```python
from build123d import *

# Parameters (mm, degrees)
SKETCH_1_R      = 1.6
SKETCH_1_R_2    = 20
SKETCH_1_R_3    = 2.1
EXTRUDE_1_DEPTH = 2
FILLET_1_R      = 3


with BuildPart() as part:
    # 草图1 → 凸台-拉伸1 (new body)
    with BuildSketch(Plane(origin=(0, 0, 0), x_dir=(1, 0, 0), z_dir=(0, 1, 0))):
        Polygon((52, 16), (-52, 16), (-52, -16), (-27.5, -16), (-27.5, -44), (27.5, -44), (27.5, -16), (52, -16), align=None)
        with Locations(Location((25, -41.5, 0), (0, 0, 270))):
            Circle(SKETCH_1_R, mode=Mode.SUBTRACT)
        with Locations(Location((-25, -41.5, 0), (0, 0, 270))):
            Circle(SKETCH_1_R, mode=Mode.SUBTRACT)
        with Locations(Location((0, -16.5, 0), (0, 0, 270))):
            Circle(SKETCH_1_R_2, mode=Mode.SUBTRACT)
        with Locations(Location((-49.1, -12.5, 0), (0, 0, 270))):
            Circle(SKETCH_1_R_3, mode=Mode.SUBTRACT)
        with Locations(Location((-49.1, 12.5, 0), (0, 0, 270))):
            Circle(SKETCH_1_R_3, mode=Mode.SUBTRACT)
        with Locations(Location((-25, 8.5, 0), (0, 0, 270))):
            Circle(SKETCH_1_R, mode=Mode.SUBTRACT)
        with Locations(Location((49.1, -12.5, 0), (0, 0, 270))):
            Circle(SKETCH_1_R_3, mode=Mode.SUBTRACT)
        with Locations(Location((25, 8.5, 0), (0, 0, 270))):
            Circle(SKETCH_1_R, mode=Mode.SUBTRACT)
        with Locations(Location((49.1, 12.5, 0), (0, 0, 270))):
            Circle(SKETCH_1_R_3, mode=Mode.SUBTRACT)
    extrude(amount=EXTRUDE_1_DEPTH)

    # 圆角1
    fillet_1_edges = [part.edges().sort_by_distance(p)[0] for p in [
        (27.5, 1, 44),
        (-27.5, 1, 44),
        (-27.5, 1, 16),
        (-52, 1, 16),
        (-52, 1, -16),
        (52, 1, -16),
        (52, 1, 16),
        (27.5, 1, 16),
    ]]
    fillet(fillet_1_edges, radius=FILLET_1_R)


solid = part.part
```
Could you check a few things on this model? Use its own coordinates, in mm. A direction names the side the tool comes from. Round coordinates to 2 decimals unless told otherwise and drop trailing zeros. Loops run counter-clockwise (first coordinate to the right, second up) from the corner with the lowest first, then second, coordinate; pieces in that order, holes last. Notation, with made-up numbers: (72.25, 21) - (98.25, 21) arc R21 cw to (98.25, 42) - close; hole circle Ø11 at (43.5, 36). An arc over 180 degrees is marked (long way). Answer in a Markdown table with one row per item. Add a question column.
(1) If we section it at C-C (y = 0.8): State how many separate pieces and enclosed holes the cut face has, plus the area to 3 significant figures.
(2) If we mould it in two halves opening along X, with no side actions, what happens to faces 1 (the face through (-47.018, 0.986, -12.773)), 2 (the face through (-23.414, 0.986, -8.708)), 3 (the face through (52, 1, 0)), 4 (the face through (40, 1, 16))? For each: pulls with the +X half, pulls with the -X half, needs draft (parallel to the pull), parting line crosses it, or undercut.
(3) If we section it at B-B (z = -8.5): Please give me the cut outline in (x, y), plus the area to 3 significant figures.
(4) I need wall thicknesses on line 1 along X through (y, z) = (1.25, -12.5); line 2 along X through (y, z) = (1.2, -8.5); line 3 along X through (y, z) = (1.75, 12). Which ranges of each line are inside material? Lowest first, please.
(5) For faces 5 (the face through (27.5, 1, 30)), 6 (the face through (-40, 1, 16)), 7 (the face through (25.07, 0.99, -10.1)), which set-ups out of +Z, -Z, +X, -X, +Y, -Y let a thin tool reach every point of the face, with its end or its side?
(6) I'm going to push flat-ended pins straight in: pin 1 (1 mm diameter, centred on y = 1, z = 32, fed in from +X); pin 2 (3 mm diameter, centred on x = -25, z = -8.5, fed in from -Y). Where does each tip first touch, or does it pass through?
(7) If we section it at A-A (x = 0): Please give me the cut outline in (y, z).
(8) If we section it at D-D (z = 33.5): Please give me the cut outline in (x, y), plus the area to 3 significant figures.
Model answer:
| question | item | result |
|---|---|---|
| 1 | separate pieces | 1 |
| 1 | enclosed holes | 9 |
| 1 | area | 3,520 mm² |
| 2 | face 1 | undercut |
| 2 | face 2 | undercut |
| 2 | face 3 | pulls with the +X half |
| 2 | face 4 | needs draft |
| 3 | outline | (-52, 0) - (-26.6, 0) - (-26.6, 2) - (-52, 2) - close; (-23.4, 0) - (23.4, 0) - (23.4, 2) - (-23.4, 2) - close; (26.6, 0) - (52, 0) - (52, 2) - (26.6, 2) - close |
| 3 | area | 195 mm² |
| 4 | line 1 | x = -52 to -51.2, -47 to 47, 51.2 to 52 |
| 4 | line 2 | x = -52 to -26.6, -23.4 to 23.4, 26.6 to 52 |
| 4 | line 3 | x = -52 to -51.14, -47.06 to -19.49, 19.49 to 47.06, 51.14 to 52 |
| 5 | face 5 | +Z, +X, +Y, -Y |
| 5 | face 6 | +Z, -X, +Y, -Y |
| 5 | face 7 | +Y, -Y |
| 6 | pin 1 | stops at x = 27.5 |
| 6 | pin 2 | passes through |
| 7 | outline | (0, -16) - (2, -16) - (2, -3.5) - (0, -3.5) - close; (0, 36.5) - (2, 36.5) - (2, 44) - (0, 44) - close |
| 8 | outline | (-27.5, 0) - (-10.54, 0) - (-10.54, 2) - (-27.5, 2) - close; (10.54, 0) - (27.5, 0) - (27.5, 2) - (10.54, 2) - close |
| 8 | area | 67.9 mm² |
